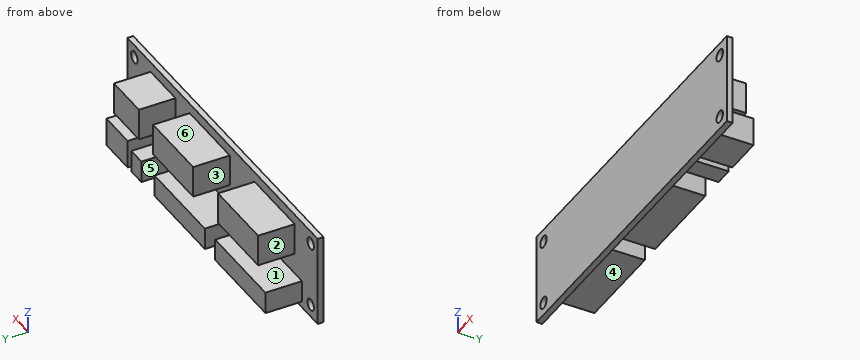
```python
from build123d import *

# Parameters (mm, degrees)
SKETCH1_W           = 95
SKETCH1_H           = 25
SKETCH1_R           = 1.6
BOSS_EXTRUDE1_DEPTH = 1.6
SKETCH2_W           = 25.078547191
SKETCH2_H           = 6
SKETCH2_W_2         = 25.078547192
SKETCH2_W_3         = 5.04587156
SKETCH2_W_4         = 20
SKETCH2_H_2         = 8.7
SKETCH2_W_5         = 10.550458716
SKETCH2_H_3         = 7.798165138
SKETCH2_W_6         = 12.457684798
BOSS_EXTRUDE2_DEPTH = 10


with BuildPart() as part:
    # Sketch1 → Boss-Extrude1 (new body)
    with BuildSketch(Plane(origin=(0, 0, 0), x_dir=(1, 0, 0), z_dir=(0, 1, 0))):
        with Locations((18, -3)):
            Rectangle(SKETCH1_W, SKETCH1_H)
        with Locations((-26, 6)):
            Circle(SKETCH1_R, mode=Mode.SUBTRACT)
        with Locations((62, 6)):
            Circle(SKETCH1_R, mode=Mode.SUBTRACT)
        with Locations((62, -12)):
            Circle(SKETCH1_R, mode=Mode.SUBTRACT)
        with Locations((-26, -12)):
            Circle(SKETCH1_R, mode=Mode.SUBTRACT)
    extrude(amount=BOSS_EXTRUDE1_DEPTH)

    # Sketch2 → Boss-Extrude2 (add)
    with BuildSketch(Plane(origin=(0, 1.6, 0), x_dir=(1, 0, 0), z_dir=(0, 1, 0))):
        with Locations((-9.162561267, 4.749179336)):
            Rectangle(SKETCH2_W, SKETCH2_H)
        with Locations((21.112668091, 4.749179336)):
            Rectangle(SKETCH2_W_2, SKETCH2_H)
        with Locations((42.747706422, 4.749179336)):
            Rectangle(SKETCH2_W_3, SKETCH2_H)
        with Locations((-8.038302451, -8.374621296)):
            Rectangle(SKETCH2_W_4, SKETCH2_H_2)
        with Locations((52.380733945, 3.850096767)):
            Rectangle(SKETCH2_W_5, SKETCH2_H_3)
        with Locations((47.682340819, -8.374621296)):
            Rectangle(SKETCH2_W_6, SKETCH2_H_2)
        with Locations((24.37710187, -8.374621296)):
            Rectangle(SKETCH2_W_4, SKETCH2_H_2)
    extrude(amount=BOSS_EXTRUDE2_DEPTH)


solid = part.part
```
Model file for the job. Use its own axes, mm. Face numbers are marked on the shaded views. A direction names the side the tool comes from. Coordinates: 2 decimals unless noted, no trailing zeros. Loops run counter-clockwise (first coordinate to the right, second up) from the corner with the lowest first, then second, coordinate; pieces in that order, holes last. Notation, with made-up numbers: M 30.5,-28.75 L 73.5,-28.75 A25 cw 73.5,-14.75 Z; hole C 44,50.25 d6. An arc over 180 degrees is marked long. Use CSV: the item, a comma, the result in double quotes. Start each with the question number.
1. Tool access for the marked faces 4, 5 and 6: list every direction of +Z, -Z, +X, -X, +Y, -Y with a clear straight run to the whole face (end or side of a thin tool).
2. Band-saw the part on D-D, the plane z = 6. List the corners of the cut face in (x, y).
3. Probe probe 1 along X at (y, z) = (1, 12); probe 2 along X at (y, z) = (10.25, 12); probe 3 along Z at (x, y) = (-26, 0.6). List the from-to ranges inside material, lowest first. Write a range as [from, to].
4. Band-saw the part on B-B, the plane y = 10.25. List the corners of the cut face in (x, z), then the cut area to 3 significant figures.
5. Flat gauge pins, fed straight in: pin 1 (4 mm diameter, centred on y = 6, z = -1.5, fed in from -X); pin 2 (3 mm diameter, centred on x = -12.5, y = 6, fed in from -Z); pin 3 (4 mm diameter, centred on y = 7.5, z = -5, fed in from +X). Where does each tip first touch, or does it go through?
6. Two-plate mould, pull along X, no slides. Class the marked faces 1, 2 and 3: pulls with the +X half, pulls with the -X half, needs draft (parallel to the pull), parting line crosses it, or undercut.
7. Band-saw the part on A-A, the plane z = -6. List the corners of the cut face in (x, y), then the cut area to 3 significant figures.
8. Band-saw the part on C-C, the plane x = -16. List the corners of the cut face in (y, z), then the cut area to 3 significant figures.
Entries:
1,face 4,"-Z, +X, -X, +Y"
1,face 5,"+Z, -Z, +Y"
1,face 6,"+Z, +X, -X, +Y"
2,outline,"M -29.5,0 L 65.5,0 L 65.5,1.6 L 53.91,1.6 L 53.91,11.6 L 41.45,11.6 L 41.45,1.6 L 34.38,1.6 L 34.38,11.6 L 14.38,11.6 L 14.38,1.6 L 1.96,1.6 L 1.96,11.6 L -18.04,11.6 L -18.04,1.6 L -29.5,1.6 Z"
3,probe 1,"x = [-29.5, -27.6], [-24.4, 60.4], [63.6, 65.5]"
3,probe 2,"x = [-18.04, 1.96], [14.38, 34.38], [41.45, 53.91]"
3,probe 3,"z = [-9.5, -7.6], [-4.4, 10.4], [13.6, 15.5]"
4,outline,"M -21.7,-7.75 L 3.38,-7.75 L 3.38,-1.75 L -21.7,-1.75 Z; M -18.04,4.02 L 1.96,4.02 L 1.96,12.72 L -18.04,12.72 Z; M 8.57,-7.75 L 33.65,-7.75 L 33.65,-1.75 L 8.57,-1.75 Z; M 14.38,4.02 L 34.38,4.02 L 34.38,12.72 L 14.38,12.72 Z; M 40.22,-7.75 L 45.27,-7.75 L 45.27,-1.75 L 40.22,-1.75 Z; M 41.45,4.02 L 53.91,4.02 L 53.91,12.72 L 41.45,12.72 Z; M 47.11,-7.75 L 57.66,-7.75 L 57.66,0.05 L 47.11,0.05 Z"
4,area,"870 mm2"
5,pin 1,"stops at x = -21.7"
5,pin 2,"stops at z = -7.75"
5,pin 3,"stops at x = 57.66"
6,face 1,"needs draft"
6,face 2,"pulls with the -X half"
6,face 3,"undercut"
7,outline,"M -29.5,0 L -27.6,0 L -27.6,1.6 L -29.5,1.6 Z; M -24.4,0 L 60.4,0 L 60.4,1.6 L 57.66,1.6 L 57.66,11.6 L 47.11,11.6 L 47.11,1.6 L 45.27,1.6 L 45.27,11.6 L 40.22,11.6 L 40.22,1.6 L 33.65,1.6 L 33.65,11.6 L 8.57,11.6 L 8.57,1.6 L 3.38,1.6 L 3.38,11.6 L -21.7,11.6 L -21.7,1.6 L -24.4,1.6 Z; M 63.6,0 L 65.5,0 L 65.5,1.6 L 63.6,1.6 Z"
7,area,"799 mm2"
8,outline,"M 0,-9.5 L 1.6,-9.5 L 1.6,-7.75 L 11.6,-7.75 L 11.6,-1.75 L 1.6,-1.75 L 1.6,4.02 L 11.6,4.02 L 11.6,12.72 L 1.6,12.72 L 1.6,15.5 L 0,15.5 Z"
8,area,"187 mm2"
